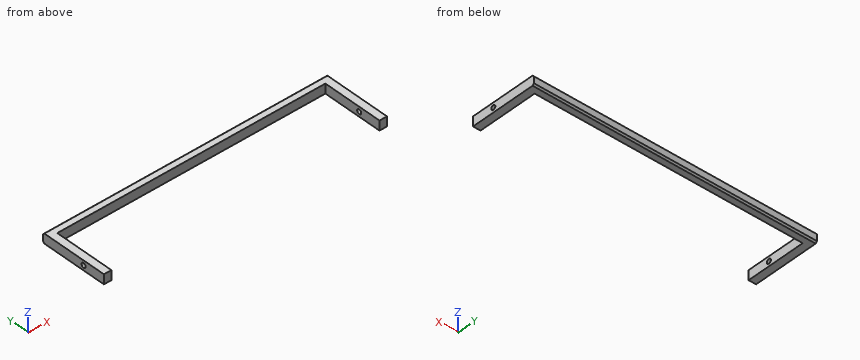
```python
from build123d import *

# Parameters (mm, degrees)
F1_DEPTH = 3.175
F3_D     = 3
F4_SIZE2 = 1
F4_SIZE  = 1
F5_SIZE2 = 1
F5_SIZE  = 1


with BuildPart() as f1:
    # F0 (on Top) → F1 (new body, symmetric)
    with BuildSketch(Plane.XY):
        Polygon((94.45, -22.5), (94.45, 22.5), (-94.45, 22.5), (-94.45, -22.5), (-89.45, -22.5), (-89.45, -15.1735553518), (-89.45, 15.1735553518), (-89.45, 17.5), (89.45, 17.5), (89.45, 15.1735553518), (89.45, -15.1735553518), (89.45, -22.5), align=None)
    extrude(amount=F1_DEPTH, both=True)

    # F3 (through all)
    with Locations(Plane(origin=(-94.45, 0, 0), x_dir=(0, -1, 0), z_dir=(-1, 0, 0))):
        with Locations((7.5, 0)):
            Hole(F3_D / 2)

    # F4
    f4_edges = [f1.edges().sort_by_distance(p)[0] for p in [
        (0, 22.5, 3.175),
    ]]
    chamfer(f4_edges, length=F4_SIZE, length2=F4_SIZE2)

    # F5
    f5_edges = [f1.edges().sort_by_distance(p)[0] for p in [
        (0, 22.5, -3.175),
    ]]
    chamfer(f5_edges, length=F5_SIZE, length2=F5_SIZE2)


solid = f1.part
```
Could you check a few things on this model? Use its own coordinates, in mm. Coordinates: 2 decimals unless noted, no trailing zeros. Order: outer loops, then holes, each group sorted by start corner. A loop starts at its lowest first (then second) coordinate and runs counter-clockwise, first axis right, second up. Notation, with made-up numbers: M 80,-17.75 L 95,-17.75 A27 cw 95,-0.75 Z; hole C 28.25,-36.75 d11. An arc over 180 degrees is marked long. Use one line per item in the form item = value. Start each with the question number.
1. Suppose I cut it at A-A on y = 1.5. Write out the boundary of the cut face in (x, z) (3 decimals).
2. Suppose I cut it at C-C on x = -23. Write out the boundary of the cut face in (y, z) (3 decimals).
3. For pin 1 (2 mm diameter, centred on x = -70, z = 1.5, fed in from -Y), with a flat end and sliding along its axis, tell me the tip position at first contact or that it passes through.
4. Please list where these lines run through material, in increasing order: line 1 (Z direction, x = 93, y = -7.5) (3 decimals); line 2 (X direction, y = -19.5, z = 0.75); line 3 (Y direction, x = -56.5, z = -0.5).
5. Suppose I cut it at B-B on z = 0. Write out the boundary of the cut face in (x, y), then the cut area to 3 significant figures.
Geometry says:
q1.outline = M -94.45,-3.175 L -89.45,-3.175 L -89.45,3.175 L -94.45,3.175 Z; M 89.45,-3.175 L 94.45,-3.175 L 94.45,3.175 L 89.45,3.175 Z
q2.outline = M 17.5,-3.175 L 21.5,-3.175 L 22.5,-2.175 L 22.5,2.175 L 21.5,3.175 L 17.5,3.175 Z
q3.pin_1 = 17.5
q4.line_1 = -3.175 to -1.5, 1.5 to 3.175
q4.line_2 = -94.45 to -89.45, 89.45 to 94.45
q4.line_3 = 17.5 to 22.5
q5.outline = M -94.45,-22.5 L -89.45,-22.5 L -89.45,-9 L -94.45,-9 Z; M -94.45,-6 L -89.45,-6 L -89.45,17.5 L 89.45,17.5 L 89.45,-6 L 94.45,-6 L 94.45,22.5 L -94.45,22.5 Z; M 89.45,-22.5 L 94.45,-22.5 L 94.45,-9 L 89.45,-9 Z
q5.area = 1,310 mm^2
